Input: part model. Units: mm. Frame: model coordinates. A direction names the side the tool comes from. Give positions to 0.01 mm unless a question says otherwise; leave off trailing zeros. Write each loop counter-clockwise with the first axis right and the second up, starting at its lowest first coordinate (ties: lowest second). Pieces come first, ordered by that corner, then holes. Notation, with made-up numbers: (29, 81) -> (46, 81) arc R22 cw to (46, 116) -> close; hole circle Ø7 at (79, 55). An arc over 180 degrees is marked (long way). Return JSON: item names as keys, results as strings. Group by question number.
Item 1: Section C-C, the plane y = -1.5. Return loops of the section in (x, z) (3 decimals).
Item 2: Set-up query: faces 4 (the face through (0, 0, 0)), 5 (the face through (0, 1.9, 5)), 6 (the face through (-0.1, -2.2, 9.525)). Return all of +Z, -Z, +X, -X, +Y, -Y with unobstructed straight access to the full face (end or side cutting, diameter ignored); none if empty.
Item 3: Line query: line 1 (Y direction, x = 0, z = -1.25); line 2 (Y direction, x = 1, z = -0.75); line 3 (Z direction, x = 0.5, y = 0). Output: solid intervals per line, ascending. Write a range as [from, to].
Item 4: Mould query, pull axis X, two halves, no side actions, for faces 1 (the face through (0, -1.9, 5)), 2 (the face through (2, -2, -7)), 3 (the face through (-1.08, -4.88, 1.15)). Classes: released by +X, released by -X, zero draft, split by the parting line, or undercut.
Item 5: Section A-A, the plane z = -1.75. Return loops of the section in (x, y).
Item 6: Section B-B, the plane x = 0. Return loops of the section in (y, z) (3 decimals).
Item 7: Pin query (flat end, axial travel): P1, Ø4, axis at y = 4, z = -1.5, coming from the -X side; P2, Ø3.5, axis at x = 0.5, z = 5.5, coming from the +Y side; P3, Ø1, axis at x = -4, z = -1.5, coming from the -Y side; P4, Ø4, axis at y = -3.5, z = 2, coming from the +X side. Return the tip coordinate at first contact, or that it passes through.
Item 8: Section D-D, the plane z = 8.5. Return loops of the section in (x, y), then the cut area to 3 significant figures.
from build123d import *

# Parameters (mm, degrees)
F0_R          = 5
F1_DEPTH      = 9.525
F1_DEPTH_BACK = 7
F4_DEPTH      = 9.526
F3_R          = 2.5
F5_DEPTH      = 7.001
F6_DEPTH      = 1.27


with BuildPart() as f1:
    # F0 (on Top) → F1 (new body, two sides)
    with BuildSketch(Plane.XY) as f1_sk:
        Circle(F0_R)
    extrude(amount=F1_DEPTH)
    extrude(f1_sk.sketch, amount=-F1_DEPTH_BACK)

    # F2 (on Top) → F4 (cut, through all)
    with BuildSketch(Plane.XY):
        with BuildLine():
            ThreePointArc((2.056696, -1.9), (2.607561, -1.02011), (2.8, 0))
            ThreePointArc((2.8, 0), (2.607561, 1.02011), (2.056696, 1.9))
            Line((2.056696, 1.9), (-2.056696, 1.9))
            ThreePointArc((-2.056696, 1.9), (-2.8, 0), (-2.056696, -1.9))
            Line((-2.056696, -1.9), (2.056696, -1.9))
        make_face()
    extrude(amount=F4_DEPTH, mode=Mode.SUBTRACT)

    # F3 (on Top) → F5 (cut, through all)
    with BuildSketch(Plane.XY):
        Circle(F3_R)
    extrude(amount=-F5_DEPTH, mode=Mode.SUBTRACT)

    # F0 (on Top) → F6 (join)
    with BuildSketch(Plane.XY):
        Circle(F0_R)
    extrude(amount=F6_DEPTH)


solid = f1.part
Answer below:
{
 "1": {"outline": "(-4.77, -7) -> (-2, -7) -> (-2, 0) -> (2, 0) -> (2, -7) -> (4.77, -7) -> (4.77, 9.525) -> (2.364, 9.525) -> (2.364, 1.27) -> (-2.364, 1.27) -> (-2.364, 9.525) -> (-4.77, 9.525) -> close"},
 "2": {"face 4": "-Z", "face 5": "+Z", "face 6": "+Z, +X, -X, +Y, -Y"},
 "3": {"line 1": "y = [-5, -2.5], [2.5, 5]", "line 2": "y = [-4.9, -2.29], [2.29, 4.9]", "line 3": "z = [0, 1.27]"},
 "4": {"face 1": "undercut", "face 2": "zero draft", "face 3": "split by the parting line"},
 "5": {"outline": "circle Ø10 at (0, 0); hole circle Ø5 at (0, 0)"},
 "6": {"outline": "(-5, -7) -> (-2.5, -7) -> (-2.5, 0) -> (2.5, 0) -> (2.5, -7) -> (5, -7) -> (5, 9.525) -> (1.9, 9.525) -> (1.9, 1.27) -> (-1.9, 1.27) -> (-1.9, 9.525) -> (-5, 9.525) -> close"},
 "7": {"P1": "stops at x = -4.58", "P2": "stops at y = 5", "P3": "stops at y = -3.57", "P4": "stops at x = 4.77"},
 "8": {"outline": "circle Ø10 at (0, 0); hole (-2.06, -1.9) -> (2.06, -1.9) arc R2.8 ccw to (2.8, 0) arc R2.8 ccw to (2.06, 1.9) -> (-2.06, 1.9) arc R2.8 ccw to start", "area": "59.0 mm2"}
}
